The listing builds one solid part. Answer for the finished solid, in the listing's coordinates (mm). Round coordinates to 2 decimals unless told otherwise and drop trailing zeros. Answer as CSV lines item,"result". Start each with the question number.
Item 1: For a pull along X with two mould halves and no side action, classify faces 1 (the cylindrical face through (25.242, -32.436, 1.479)), 2 (the flat face through (-1.6, 17, 1.6)), 3 (the cylindrical face through (-13.35, -38.87, 1.48)) as pulls with the +X half, pulls with the -X half, needs draft (parallel to the pull), parting line crosses it, or undercut.
Item 2: A cutting plane is placed at A-A on y = 34. State how many separate pieces and enclosed holes the cut face has, and give its area (3 significant figures).
Item 3: Flat-ended cylindrical pins translate along their axes: pin 1 (1 mm diameter, centred on y = 21, z = 2, fed in from +X); pin 2 (1 mm diameter, centred on y = -21.5, z = 2, fed in from -X); pin 3 (1 mm diameter, centred on y = -23, z = 1.5, fed in from +X). Find the tip coordinate at first contact, or state that the pin passes through.
Item 4: Straight lines are drawn through the part: line 1 along X through (y, z) = (28, 0.2); line 2 along Z through (x, y) = (32, -12.5); line 3 along X through (y, z) = (-2, -0.55). For each, find the intervals that lie inside material, in ascending order. Write a range as [from, to].
```python
from build123d import *

# Parameters (mm, degrees)
SKETCH_1_R      = 26
EXTRUDE_1_DEPTH = 3
SKETCH_2_R      = 22.8
EXTRUDE_2_DEPTH = 3
FILLET_8_R      = 17


with BuildPart() as part:
    # Sketch 1 → Extrude 1 (new body)
    with BuildSketch(Plane.XY):
        with BuildLine():
            ThreePointArc((-5.5, 40.730332677), (-6.779718382, 40.536963609), (-8.052713795, 40.303396886))
            add(Edge.make_bspline(
                [(-18.42711223, 36.737603826), (-9.565846889, 27.871779004), (-8.052713795, 40.303396886)],
                knots=[0, 0, 0, 1, 1, 1], degree=2))
            ThreePointArc((-18.42711223, 36.737603826), (-19.574705107, 36.139188148), (-20.702887125, 35.504935779))
            add(Edge.make_bspline(
                [(-29.357360924, 28.763785557), (-18.097494767, 23.255583732), (-20.702887125, 35.504935779)],
                knots=[0, 0, 0, 1, 1, 1], degree=2))
            ThreePointArc((-29.357360924, 28.763785557), (-30.2484688, 27.825170893), (-31.109581398, 26.858963965))
            add(Edge.make_bspline(
                [(-37.106284036, 17.672964807), (-24.667998276, 16.119285114), (-31.109581398, 26.858963965)],
                knots=[0, 0, 0, 1, 1, 1], degree=2))
            ThreePointArc((-37.106284036, 17.672964807), (-37.644341546, 16.49586462), (-38.145069811, 15.302406645))
            add(Edge.make_bspline(
                [(-40.834165508, 4.667004096), (-28.565341408, 7.236211838), (-38.145069811, 15.302406645)],
                knots=[0, 0, 0, 1, 1, 1], degree=2))
            ThreePointArc((-40.834165508, 4.667004096), (-40.960865773, 3.378975456), (-41.046948028, 2.087596124))
            add(Edge.make_bspline(
                [(-40.137031541, -8.844698925), (-29.367186562, -2.431017271), (-41.046948028, 2.087596124)],
                knots=[0, 0, 0, 1, 1, 1], degree=2))
            ThreePointArc((-40.137031541, -8.844698925), (-39.83864462, -10.104078129), (-39.500752518, -11.353437829))
            add(Edge.make_bspline(
                [(-35.090427416, -21.397941578), (-26.986641373, -11.834807939), (-39.500752518, -11.353437829)],
                knots=[0, 0, 0, 1, 1, 1], degree=2))
            ThreePointArc((-35.090427416, -21.397941578), (-34.399288162, -22.492198068), (-33.674037554, -23.564150627))
            add(Edge.make_bspline(
                [(-26.241230996, -31.632385237), (-21.68167485, -19.95611353), (-33.674037554, -23.564150627)],
                knots=[0, 0, 0, 1, 1, 1], degree=2))
            ThreePointArc((-26.241230996, -31.632385237), (-25.232235072, -32.442939344), (-24.198218116, -33.221322069))
            add(Edge.make_bspline(
                [(-14.548390024, -38.438969129), (-14.027162432, -25.91486457), (-24.198218116, -33.221322069)],
                knots=[0, 0, 0, 1, 1, 1], degree=2))
            ThreePointArc((-14.548390024, -38.438969129), (-13.330877794, -38.877984737), (-12.10014627, -39.278447783))
            add(Edge.make_bspline(
                [(-1.27900525, -41.080094274), (-4.85258931, -29.065337922), (-12.10014627, -39.278447783)],
                knots=[0, 0, 0, 1, 1, 1], degree=2))
            ThreePointArc((-1.27900525, -41.080094274), (0.015086944, -41.099997231), (1.309164177, -41.079144212))
            add(Edge.make_bspline(
                [(12.128979588, -39.269553781), (4.84783716, -29.066130916), (1.309164177, -41.079144212)],
                knots=[0, 0, 0, 1, 1, 1], degree=2))
            ThreePointArc((12.128979588, -39.269553781), (13.359416777, -38.868187292), (14.576606372, -38.428277956))
            add(Edge.make_bspline(
                [(24.222601287, -33.203547806), (14.022925251, -25.917157617), (14.576606372, -38.428277956)],
                knots=[0, 0, 0, 1, 1, 1], degree=2))
            ThreePointArc((24.222601287, -33.203547806), (25.256046509, -32.424406158), (26.264447087, -31.613111508))
            add(Edge.make_bspline(
                [(33.691328284, -23.53942222), (21.678411803, -19.959658145), (26.264447087, -31.613111508)],
                knots=[0, 0, 0, 1, 1, 1], degree=2))
            ThreePointArc((33.691328284, -23.53942222), (34.415791714, -22.466937501), (35.106127425, -21.3721739))
            add(Edge.make_bspline(
                [(39.509077087, -11.324434984), (26.984706061, -11.839220006), (35.106127425, -21.3721739)],
                knots=[0, 0, 0, 1, 1, 1], degree=2))
            ThreePointArc((39.509077087, -11.324434984), (39.846051872, -10.074827555), (40.143514129, -8.815229627))
            add(Edge.make_bspline(
                [(41.045404341, 2.117730498), (29.366788706, -2.435818675), (40.143514129, -8.815229627)],
                knots=[0, 0, 0, 1, 1, 1], degree=2))
            ThreePointArc((41.045404341, 2.117730498), (40.958374033, 3.409046284), (40.830728186, 4.696981559))
            add(Edge.make_bspline(
                [(38.13382515, 15.330407021), (28.566524123, 7.231541404), (40.830728186, 4.696981559)],
                knots=[0, 0, 0, 1, 1, 1], degree=2))
            ThreePointArc((38.13382515, 15.330407021), (37.632220833, 16.523497062), (37.093299291, 17.700201912))
            add(Edge.make_bspline(
                [(31.089854296, 26.881796068), (24.670633395, 16.115251764), (37.093299291, 17.700201912)],
                knots=[0, 0, 0, 1, 1, 1], degree=2))
            ThreePointArc((31.089854296, 26.881796068), (30.228032583, 27.847370544), (29.336235855, 28.785330741))
            add(Edge.make_bspline(
                [(20.676815321, 35.520125397), (18.101296735, 23.252624541), (29.336235855, 28.785330741)],
                knots=[0, 0, 0, 1, 1, 1], degree=2))
            ThreePointArc((20.676815321, 35.520125397), (19.548167965, 36.153549331), (18.400136066, 36.751122333))
            add(Edge.make_bspline(
                [(8.023122571, 40.309297987), (9.570403703, 27.870214648), (18.400136066, 36.751122333)],
                knots=[0, 0, 0, 1, 1, 1], degree=2))
            ThreePointArc((8.023122571, 40.309297987), (6.749956027, 40.541930068), (5.470096027, 40.734359569))
            add(Edge.make_bspline(
                [(-5.5, 40.730332677), (0.001292393, 30.277504211), (5.470096027, 40.734359569)],
                knots=[0, 0, 0, 1, 1, 1], degree=2))
        make_face()
        Circle(SKETCH_1_R, mode=Mode.SUBTRACT)
    extrude(amount=EXTRUDE_1_DEPTH)



with BuildPart() as body_2:
    # Sketch 2 → Extrude 2 (new body)
    with BuildSketch(Plane(origin=(0, 0, 1.6), x_dir=(-1, 0, 0), z_dir=(0, 0, -1))):
        Circle(SKETCH_2_R)
        with BuildLine():
            ThreePointArc((16.687373481, -6.747708226), (15.588457268, 9), (2.5, 17.82554347))
            ThreePointArc((2.5, 17.82554347), (0, 16.199996074), (-2.5, 17.82554347))
            ThreePointArc((-2.5, 17.82554347), (-15.588457268, 9), (-16.687373481, -6.747708226))
            ThreePointArc((-16.687373481, -6.747708226), (-14.029608141, -8.099998037), (-14.187373481, -11.077835244))
            ThreePointArc((-14.187373481, -11.077835244), (0, -18), (14.187373481, -11.077835244))
            ThreePointArc((14.187373481, -11.077835244), (14.029608141, -8.099998037), (16.687373481, -6.747708226))
        make_face(mode=Mode.SUBTRACT)
    extrude(amount=EXTRUDE_2_DEPTH)


with BuildPart() as part_1:
    add(part.part)

    add(body_2.part)  # Revolve 1 merges body 2
    # Sketch 18 → Revolve 1 (revolve)
    with BuildSketch(Plane(origin=(0, 0, 0), x_dir=(1, 0, 0), z_dir=(0, 1, 0))):
        Polygon((26, -3), (22.8, -1.6), (22.8, 1.4), (26, 0), align=None)
    revolve(axis=Axis((0, 0, 0), (0, 0, -1)))

    # Fillet 8
    # the kernel refuses this fillet: 17 mm, written as the material it takes off along each edge
    with BuildSketch(Plane(origin=(0, 0, 3), x_dir=(1, 0, 0), z_dir=(0, -1, 0))) as fillet_8_piece_1_section:
        with BuildLine():
            CenterArc((26 + FILLET_8_R * 0.209178456653, -FILLET_8_R), FILLET_8_R, 90, 23.629377731)
            Line((26 - FILLET_8_R * 0.191640377366, -FILLET_8_R * 0.0838426650978), (26, 0))
            Line((26, 0), (26 + FILLET_8_R * 0.209178456653, 0))
        make_face()
    fillet_8_piece_1 = revolve(axis=Axis((0, 0, 3), (0, 0, 1)), mode=Mode.PRIVATE)
    fillet_8_piece_1 = split(fillet_8_piece_1, bisect_by=Plane(origin=(-26.08987022, 0, 1.6), z_dir=(0, 0, 1)), keep=Keep.TOP, mode=Mode.PRIVATE)
    add(fillet_8_piece_1, mode=Mode.SUBTRACT)


solid = part_1.part
```
Geometry says:
1,face 1,"pulls with the +X half"
1,face 2,"undercut"
1,face 3,"pulls with the -X half"
2,separate pieces,"3"
2,enclosed holes,"0"
2,area,"93.1 mm^2"
3,pin 1,"stops at x = 28.93"
3,pin 2,"stops at x = -35.09"
3,pin 3,"stops at x = 34.39"
4,line 1,"x = [-30.09, -27.65], [-21.23, 21.23], [27.59, 30.09]"
4,line 2,"z = [0, 3]"
4,line 3,"x = [-24.66, -17.89], [17.89, 24.66]"
